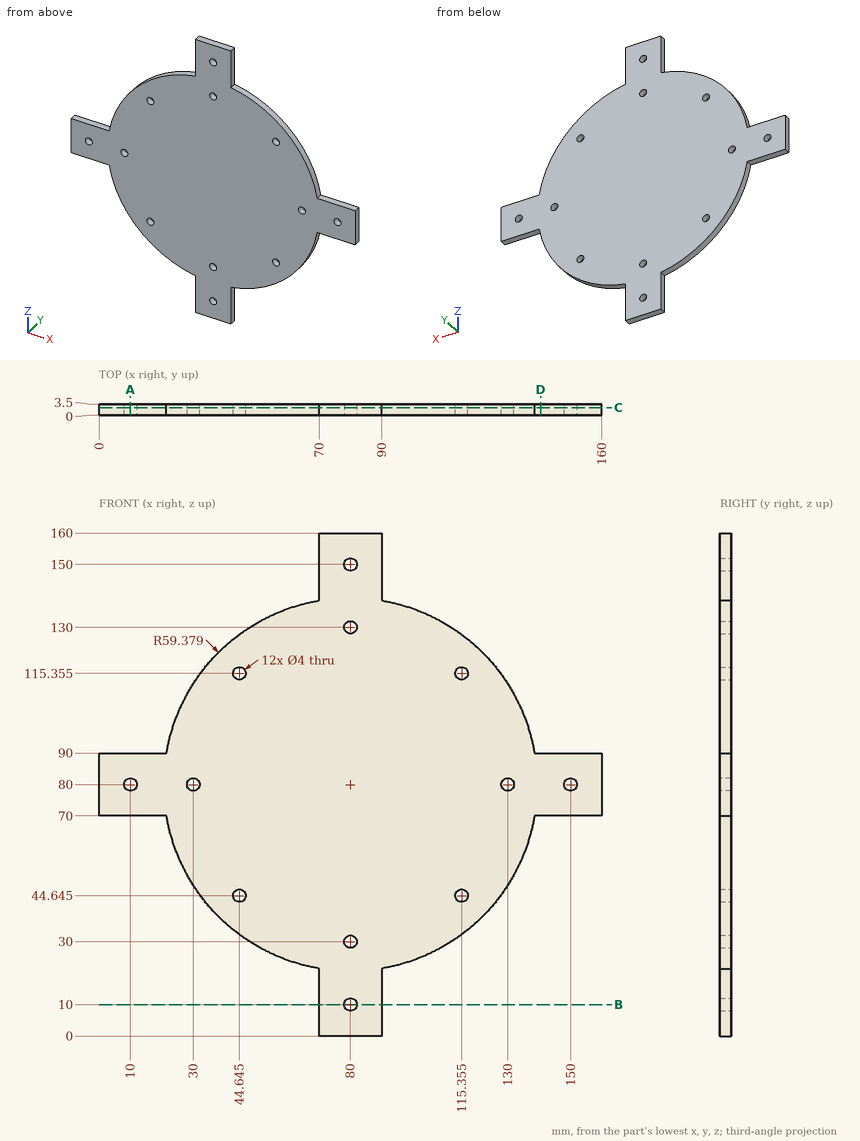
Verification items for this drawing (mm, ordinates from the low corner). Round coordinates to 2 decimals unless told otherwise and drop trailing zeros. Write each loop counter-clockwise with the first axis right and the second up, starting at its lowest first coordinate (ties: lowest second). Pieces come first, ordered by that corner, then holes. Notation, with made-up numbers: (-7.75, 73) - (0.25, 73) arc R15 ccw to (0.25, 78) - close; hole circle Ø6 at (42.5, 73). An arc over 180 degrees is marked (long way). One line per item, written item: value.
1. Cross-section at A-A on x = 10. Record the boundary of the cut face in (y, z), and give its area (3 significant figures).
The answers:
outline: (0, 70) - (3.5, 70) - (3.5, 78) - (0, 78) - close; (0, 82) - (3.5, 82) - (3.5, 90) - (0, 90) - close
area: 56.0 mm^2
2. Depth check by flat-ended pin: pin 1 Ø1 at (y, z) = (1, 12.5) entering from +X; pin 2 Ø1.8 at (x, y) = (152, 1) entering from +Z; pin 3 Ø1 at (x, y) = (7, 2) entering from -Z. Enter the tip coordinate at first touch or a pass-through.
The answers:
pin 1: stops at x = 90
pin 2: stops at z = 90
pin 3: stops at z = 70
3. Cross-section at C-C on y = 2.35. Give the number of separate pieces and of enclosed holes in the cut face, and give its area (3 significant figures).
The answers:
separate pieces: 1
enclosed holes: 12
area: 12,600 mm^2
4. Cross-section at D-D on x = 140.5. Record the boundary of the cut face in (y, z), and give its area (3 significant figures).
The answers:
outline: (0, 70) - (3.5, 70) - (3.5, 90) - (0, 90) - close
area: 70.0 mm^2
5. Scan lines: L1, parallel to Z at x = 80, y = 1.3; L2, parallel to X at y = 1.15, z = 10. Record each from-to range of solid material in increasing order.
The answers:
L1: z = 0 to 8, 12 to 28, 32 to 128, 132 to 148, 152 to 160
L2: x = 70 to 78, 82 to 90
6. Cross-section at B-B on z = 10. Record the boundary of the cut face in (x, y).
The answers:
outline: (70, 0) - (78, 0) - (78, 3.5) - (70, 3.5) - close; (82, 0) - (90, 0) - (90, 3.5) - (82, 3.5) - close
